For this review, take the finished solid that the model builds, in its own axes (mm). Face numbers are marked on the shaded views. A direction names the side the tool comes from. Give positions to 0.01 mm unless a question says otherwise; leave off trailing zeros. Loops run counter-clockwise (first coordinate to the right, second up) from the corner with the lowest first, then second, coordinate; pieces in that order, holes last. Notation, with made-up numbers: (74, 32) - (114, 32) arc R26 cw to (114, 62) - close; hole circle Ø6 at (11.5, 13.25). An arc over 180 degrees is marked (long way). Put each result on its own line as item: value. Start each with the question number.
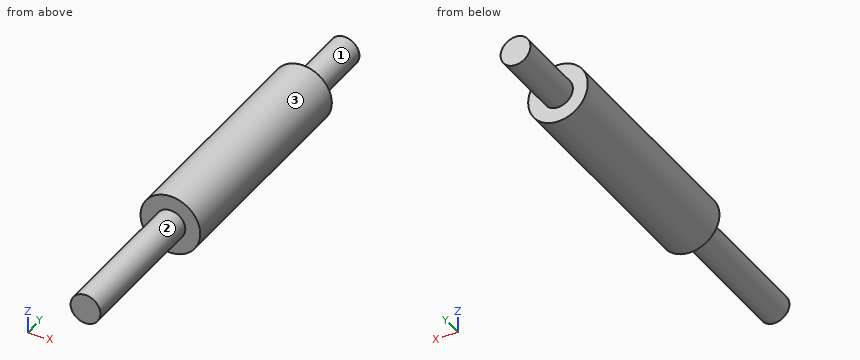
from build123d import *

# Parameters (mm, degrees)
SKETCH1_R                = 4
SKETCH1_R_2              = 2
BOSS_EXTRUDE1_DEPTH      = 31
SKETCH1_4_R              = 2
BOSS_EXTRUDE2_DEPTH      = 41
BOSS_EXTRUDE2_DEPTH_BACK = 20


with BuildPart() as part:
    # Sketch1 → Boss-Extrude1 (new body)
    with BuildSketch(Plane(origin=(0, 0, 0), x_dir=(1, 0, 0), z_dir=(0, 1, 0))):
        Circle(SKETCH1_R)
        Circle(SKETCH1_R_2, mode=Mode.SUBTRACT)
        Circle(SKETCH1_R_2)
    extrude(amount=BOSS_EXTRUDE1_DEPTH)

    # Sketch1_4 → Boss-Extrude2 (add, two sides)
    with BuildSketch(Plane(origin=(0, 0, 0), x_dir=(1, 0, 0), z_dir=(0, 1, 0))) as boss_extrude2_sk:
        Circle(SKETCH1_4_R)
    extrude(amount=BOSS_EXTRUDE2_DEPTH)
    extrude(boss_extrude2_sk.sketch, amount=-BOSS_EXTRUDE2_DEPTH_BACK)


solid = part.part
1) Machinability: for the marked faces 1, 2 and 3, which of the approach directions +Z, -Z, +X, -X, +Y, -Y give a long, thin tool a straight path to every point of the face, cutting with its end or side? Answer none if there is none.
2) Insertion check: P1, Ø1, axis at y = -6, z = -1.5, coming from the +X side; P2, Ø2, axis at x = -2.5, y = -13.5, coming from the -Z side. Each pin has a flat end and moves straight along its axis. Give the tip position at first contact, or say it passes through.
3) Take a section at B-B on x = 0. State the section outline as (y, z) points.
4) Take a section at C-C on y = -2. State the section outline as (x, z) points, and give its area (3 significant figures).
5) Wall thickness on probe 1 along X at (y, z) = (14, -0.25); probe 2 along Y at (x, z) = (2.25, -1); probe 3 along Z at (x, y) = (2.5, 26.5): over which ranges is each line inside the solid? List them lowest first.
6) Take a section at A-A on z = 0. State the section outline as (x, y) points, and give its area (3 significant figures).
7) Take a section at D-D on y = 21. State the section outline as (x, z) points, and give its area (3 significant figures).
Answers follow:
1. face 1: +Y
1. face 2: -Y
1. face 3: +Y, -Y
2. P1: x = 1.73
2. P2: z = -1.32
3. outline: (-20, -2) - (0, -2) - (0, -4) - (31, -4) - (31, -2) - (41, -2) - (41, 2) - (31, 2) - (31, 4) - (0, 4) - (0, 2) - (-20, 2) - close
4. outline: circle Ø4 at (0, 0)
4. area: 12.6 mm2
5. probe 1: -3.99 to 3.99
5. probe 2: 0 to 31
5. probe 3: -3.12 to 3.12
6. outline: (-4, 0) - (-2, 0) - (-2, -20) - (2, -20) - (2, 0) - (4, 0) - (4, 31) - (2, 31) - (2, 41) - (-2, 41) - (-2, 31) - (-4, 31) - close
6. area: 368 mm2
7. outline: circle Ø8 at (0, 0)
7. area: 50.3 mm2
